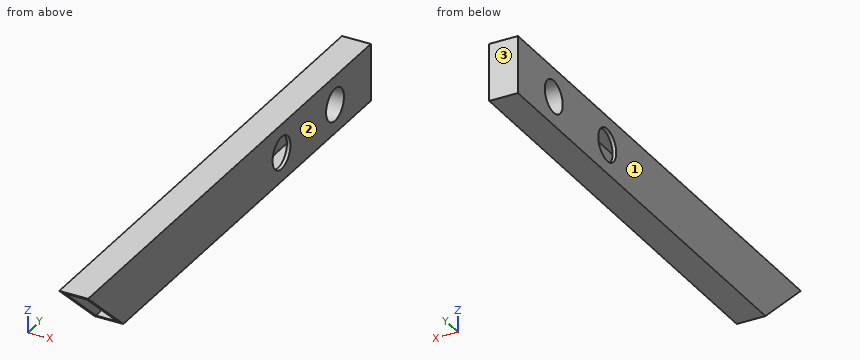
Autodesk Inventor part; units mm, degrees
ref_plane "YZ Plane" through (0, 0, 0) normal (1, 0, 0) x (0, 1, 0)
ref_plane "XZ Plane" through (0, 0, 0) normal (0, 1, 0) x (-1, 0, 0)
ref_plane "XY Plane" through (0, 0, 0) normal (0, 0, 1) x (1, 0, 0)
sketch "Sketch1" plane through (0, 0, 0) normal (0, 1, 0) x (-1, 0, 0)
  line L0 (0, 0) -> (25.4, 0)
  line L1 (25.4, 0) -> (25.4, -50.8)
  line L2 (25.4, -50.8) -> (0, -50.8)
  line L3 (0, -50.8) -> (0, 0)
  line L4 (22.225, -3.175) -> (3.175, -3.175)
  line L5 (3.175, -3.175) -> (3.175, -47.625)
  line L6 (3.175, -47.625) -> (22.225, -47.625)
  line L7 (22.225, -47.625) -> (22.225, -3.175)
  dimension "d0" = 25.4
  dimension "d1" = 50.8
  dimension "d2" = 3.175
extrude "Extrusion1" add sketch "Sketch1" along normal blind 106.553
sketch "Sketch4" plane through (0, 0, 0) normal (0, -1, 0) x (1, 0, 0)
  line L0 (-22.225, -47.625) -> (-22.225, -3.175)
  line L1 (-22.225, -3.175) -> (-3.175, -3.175)
  line L2 (-3.175, -3.175) -> (-3.175, -47.625)
  line L3 (-3.175, -47.625) -> (-22.225, -47.625)
  line L4 (0, 0) -> (-25.4, 0)
  line L5 (-25.4, 0) -> (-25.4, -50.8)
  line L6 (-25.4, -50.8) -> (0, -50.8)
  line L7 (0, -50.8) -> (0, 0)
extrude "Extrusion2" add sketch "Sketch4" along normal blind 254
sketch "Sketch5" plane through (0, 106.553, 0) normal (1, 0, 0) x (0, 0, -1)
  line L0 (50.8, 0) -> (50.8, -360.553)
  line L1 (0, 0) -> (50.8, 0)
  line L2 (0, -360.553) -> (0, 0)
  line L3 (50.8, -360.553) -> (0, -360.553)
  line L4 (0, -360.553) -> (23.3209, -360.553)
  line L5 (0, -360.553) -> (50.8, -360.553)
  line L6 (0, -360.553) -> (9.2137, -369.7667)
  line L7 (0, -360.553) -> (9.2137, -360.553)
  line L8 (9.2137, -360.553) -> (9.2137, -369.7667)
  line L9 (9.2137, -369.7667) -> (0, -369.7667)
  line L10 (0, -369.7667) -> (0, -360.553)
  line L11 (0, -369.7667) -> (0, -378.9805)
  line L12 (0, -378.9805) -> (50.8, -322.5614)
  line L13 (50.8, 0) -> (50.8, -360.553)
  line L14 (50.8, -322.5614) -> (0, -322.5614)
  line L15 (0, -322.5614) -> (0, -378.9805)
  line L16 (0, -378.9805) -> (50.8, -378.9805)
  line L17 (50.8, -378.9805) -> (50.8, -322.5614)
  point P0 (0, -106.553)
  dimension "d22" = 13.0302
  dimension "d23" = 45
  dimension "d24" = 48
extrude "Extrusion3" add sketch "Sketch5" against normal blind 25.4 contours L12 L3 L2 L14 | L12 L8 L3 | L8 L12 L6 L3 | L6 L12 L9 L10 | L11 L9 L12
extrude "Extrusion4" cut sketch "Sketch5" against normal blind 25.4 contours L0 L3 L12 | L17 L16 L12 L9 L8 L3 | L8 L6 L12 | L9 L12 L6
sketch "Sketch6" plane through (0, 106.553, 0) normal (0, 1, 0) x (1, 0, 0)
  line L0 (-22.225, 3.175) -> (-22.225, 47.625)
  line L1 (-3.175, 3.175) -> (-22.225, 3.175)
  line L2 (-3.175, 47.625) -> (-3.175, 3.175)
  line L3 (-22.225, 47.625) -> (-3.175, 47.625)
  point P0 (0, 0)
extrude "Extrusion5" cut sketch "Sketch6" against normal through all
sketch "Sketch8" plane through (0, 106.553, 0) normal (0, 1, 0) x (1, 0, 0)
  line L0 (0, 50.8) -> (-25.4, 50.8)
  line L1 (-25.4, 50.8) -> (-25.4, 0)
  line L2 (0, 50.8) -> (-25.4, 50.8)
  line L3 (-25.4, 50.8) -> (-25.4, 0)
  line L4 (-25.4, 0) -> (0, 0)
  line L5 (0, 0) -> (0, 50.8)
  line L6 (-3.175, 47.625) -> (-22.225, 47.625)
  line L7 (-22.225, 47.625) -> (-22.225, 3.175)
  line L8 (-22.225, 3.175) -> (-3.175, 3.175)
  line L9 (-3.175, 3.175) -> (-3.175, 47.625)
  dimension "d39" = 3.175
extrude "Extrusion6" add sketch "Sketch8" along normal blind 72.6948 contours L5 L4 L1 L0 | L9 L8 L7 L6
sketch "Sketch9" plane through (-25.4, -272.4275, 0) normal (-1, 0, 0) x (0, 0, 1)
  circle A0 centre (-25.4, 394.5507) radius 14.2875
  line L0 (-50.8, 451.6753) -> (0, 451.6753)
  point P0 (0, 272.4275)
  point P1 (-25.4, 340.8805)
  dimension "d44" = 28.575
  dimension "d45" = 57.1246
extrude "Extrusion7" cut sketch "Sketch9" against normal blind 158.75
sketch "Sketch10" plane through (-25.4, -272.4275, 0) normal (-1, 0, 0) x (0, 0, 1)
  circle A0 centre (-25.4, 309.1305) radius 14.2875
  point P0 (0, 272.4275)
  point P1 (-25.4, 264.6805)
  dimension "d48" = 28.575
  dimension "d49" = 44.45
extrude "Extrusion8" cut sketch "Sketch10" against normal blind 158.75
properties part number "StorageSupport.ver2-1111-2021" material "Aluminum 6061"
Here's how the part is built. I have some questions about the finished solid (model axes, mm). Face numbers are marked on the shaded views. Round coordinates to 2 decimals unless told otherwise and drop trailing zeros. Loops run counter-clockwise (first coordinate to the right, second up) from the corner with the lowest first, then second, coordinate; pieces in that order, holes last.
1. Suppose I cut it at A-A, the plane y = -25. Please give me the cut outline in (x, z) (3 decimals), and give its area (3 significant figures).
Answers:
outline: (-25.4, -50.8) - (0, -50.8) - (0, 0) - (-25.4, 0) - close; hole (-22.225, -47.625) - (-3.175, -47.625) - (-3.175, -3.175) - (-22.225, -3.175) - close
area: 444 mm2
2. Will these pins go through, and if not, where does the flat tip stop? pin 1 (5.5 mm diameter, centred on x = -9, y = -121.5, fed in from +Z); pin 2 (9.5 mm diameter, centred on x = -15, z = -22.5, fed in from -Y); pin 3 (17 mm diameter, centred on y = 36.703, z = -25.4, fed in from +X); pin 4 (8 mm diameter, centred on x = -5.5, z = -38, fed in from -Y).
Answers:
pin 1: stops at z = 0
pin 2: stops at y = 106.55
pin 3: passes through
pin 4: stops at y = -233.84
3. Suppose I cut it at B-B, the plane z = -20.5. Please give me the cut outline in (x, y) (3 decimals).
Answers:
outline: (-25.4, -249.66) - (-22.225, -249.66) - (-22.225, 23.282) - (-25.4, 23.282) - close; (-25.4, 50.124) - (-22.225, 50.124) - (-22.225, 106.553) - (-3.175, 106.553) - (-3.175, 50.124) - (0, 50.124) - (0, 108.702) - (-25.4, 108.702) - close; (-25.4, 135.544) - (0, 135.544) - (0, 179.248) - (-25.4, 179.248) - close; (-3.175, -249.66) - (0, -249.66) - (0, 23.282) - (-3.175, 23.282) - close
4. Suppose I cut it at C-C, the plane x = -17.75. Please give me the cut outline in (y, z) (1 decimal).
Answers:
outline: (-272.4, 0) - (-268.9, -3.2) - (106.6, -3.2) - (106.6, -47.6) - (-219.5, -47.6) - (-216, -50.8) - (179.2, -50.8) - (179.2, 0) - close; hole circle Ø28.6 at (122.1, -25.4)
5. Thinking about a two-plate mould opening in X: for the marked faces 1, 2 and 3, which applies, released by +X, released by -X, zero draft, split by the parting line, or undercut?
Answers:
face 1: released by -X
face 2: released by +X
face 3: zero draft
6. If I drill on probe 1 along Z at (x, y) = (-10, -172.5) (3 decimals); probe 2 along X at (y, z) = (-89, -37.5) (3 decimals); probe 3 along Y at (x, z) = (-10, -25.4), over which ranges is the centre line in solid material (lowest first)?
Answers:
probe 1: z = -50.8 to -47.625, -3.175 to 0
probe 2: x = -25.4 to -22.225, -3.175 to 0
probe 3: y = 106.55 to 107.84, 136.41 to 179.25
